Autodesk Fusion 360 part; units mm, degrees
sketch "Sketch1" plane through (0, 0, 0) normal (0, 0, 1) x (1, 0, 0)
  line L0 (20.1643, 5) -> (80.1643, 5)
  line L1 (80.1643, 5) -> (80.1643, 43)
  line L2 (80.1643, 43) -> (20.1643, 43)
  line L3 (20.1643, 43) -> (20.1643, 5)
  line L4 (24.1483, 34.1483) -> (36.6483, 34.1483)
  line L5 (36.6483, 34.1483) -> (36.6483, 10.1483)
  line L6 (36.6483, 10.1483) -> (24.1483, 10.1483)
  line L7 (24.1483, 10.1483) -> (24.1483, 34.1483)
  circle A0 centre (74.6483, 29.6742) radius 1.75
  circle A1 centre (74.6483, 13.1742) radius 1.75
  line L8 (74.6483, 29.6742) -> (74.6483, 13.1742)
  line L9 (74.6483, 21.4242) -> (52.6483, 21.4242)
  circle A2 centre (52.6483, 21.4242) radius 1.75
  line L10 (95, 35) -> (105, 35)
  line L11 (105, 35) -> (105, 25)
  line L12 (105, 25) -> (95, 25)
  line L13 (95, 25) -> (95, 35)
  circle A3 centre (100, 30) radius 1.75
  circle A4 centre (30.3983, 8.1483) radius 1.75
  line L14 (24.1483, 22.1483) -> (9, 22.1483) construction
  circle A5 centre (30.3983, 36.1483) radius 1.75
  line L15 (80.1643, 27.7253) -> (80.1643, 24.8327)
  line L16 (36.6483, 24.8327) -> (36.6483, 27.7253)
  dimension "d1" = 60
  dimension "d2" = 38
  dimension "d3" = 24
  dimension "d4" = 12.5
  dimension "d6" = 3.5
  dimension "d7" = 16.5
  dimension "d8" = 3.5
  dimension "d9" = 38
  dimension "d10" = 22
  dimension "d11" = 3.5
  dimension "d12" = 3.5
  dimension "d16" = 3.5
  dimension "d17" = 2
extrude "Extrude1" add sketch "Sketch1" along normal blind 5 contours L0 L1 L2 L3 L15 | L10 L11 L12 L13 | A4 | A5 makes body 1 at (41.3983, 21.907, 0) makes body 2 at (99.9564, 33.915, 0)
extrude "Extrude2" cut sketch "Sketch1" along normal blind 100 contours A4 | A5 bodies 1
delete_body "RemoveBody1" bodies 2
The listing builds one solid part. Answer for the finished solid, in the listing's coordinates (mm). A direction names the side the tool comes from. Round coordinates to 2 decimals unless told otherwise and drop trailing zeros. Loops run counter-clockwise (first coordinate to the right, second up) from the corner with the lowest first, then second, coordinate; pieces in that order, holes last. Notation, with made-up numbers: M 1,70 L 25,70 A23 ccw 25,107 Z; hole C -23.5,83.25 d5. An arc over 180 degrees is marked long. Write each question's results on one line, items separated by ' | '. Start each with the question number.
1) This flat-tipped pin is pushed along its axis until it touches: pin 1 (3 mm diameter, centred on x = 30.4, y = 8.15, fed in from +Z). Where does it stop, or does it pass through?
2) Find section C-C on x = 75.5. Write down the section's boundary in (y, z).
3) Find section A-A on x = 34. Write down the section's boundary in (y, z).
4) Which of the six approach directions +Z, -Z, +X, -X, +Y, -Y give full straight-line access (tool end or side, diameter ignored) to faces 1 (the flat face through (30, 34.148, 2)), 2 (the flat face through (80.164, 24, 2))?
5) Straight lines are drawn through the part: probe 1 along Y at (x, z) = (34, 4.2); probe 2 along Y at (x, z) = (30, 4.4); probe 3 along X at (y, z) = (31, 0.55). For each, find the intervals that lie inside material, in ascending order.
6) Find section B-B on y = 26.5. Write down the section's boundary in (x, z).
7) Determine the mould class of faces 3 (the cylindrical face through (74.269, 31.383, 2.465)), 4 (the flat face through (20.164, 24, 2)), 5 (the flat face through (56, 24, 5)), 6 (the flat face through (30, 10.148, 2)) for opening direction X: pulls with the +X half, pulls with the -X half, needs draft (parallel to the pull), parting line crosses it, or undercut.
8) Find section D-D on z = 2.05. Write down the section's boundary in (x, y), plus the area to 3 significant figures.
Final values:
1) pin 1: through
2) outline: M 5,0 L 11.65,0 L 11.65,5 L 5,5 Z; M 14.7,0 L 28.15,0 L 28.15,5 L 14.7,5 Z; M 31.2,0 L 43,0 L 43,5 L 31.2,5 Z
3) outline: M 5,0 L 10.15,0 L 10.15,5 L 5,5 Z; M 34.15,0 L 43,0 L 43,5 L 34.15,5 Z
4) face 1: +Z, -Z | face 2: +Z, -Z, +X, +Y, -Y
5) probe 1: 5 to 10.15, 34.15 to 43 | probe 2: 5 to 6.44, 9.85 to 10.15, 34.15 to 34.44, 37.85 to 43 | probe 3: 20.16 to 24.15, 36.65 to 73.51, 75.79 to 80.16
6) outline: M 20.16,0 L 24.15,0 L 24.15,5 L 20.16,5 Z; M 36.65,0 L 80.16,0 L 80.16,5 L 36.65,5 Z
7) face 3: undercut | face 4: pulls with the -X half | face 5: needs draft | face 6: undercut
8) outline: M 20.16,5 L 80.16,5 L 80.16,43 L 20.16,43 Z; hole M 24.15,10.15 L 36.65,10.15 L 36.65,34.15 L 24.15,34.15 Z; hole C 30.4,8.15 d3.5; hole C 30.4,36.15 d3.5; hole C 52.65,21.42 d3.5; hole C 74.65,13.17 d3.5; hole C 74.65,29.67 d3.5 | area: 1,930 mm²
